Model file for the job. Use its own axes, mm. Face numbers are marked on the shaded views. A direction names the side the tool comes from. Coordinates: 2 decimals unless noted, no trailing zeros. Loops run counter-clockwise (first coordinate to the right, second up) from the corner with the lowest first, then second, coordinate; pieces in that order, holes last. Notation, with made-up numbers: M 73,10 L 106,10 A9 cw 106,25 Z; hole C -39.5,9.25 d9. An arc over 180 degrees is marked long. Write item = value, one per line. Start each with the question number.
from build123d import *

# Parameters (mm, degrees)
BOSS_EXTRUDE1_DEPTH = 127
BOSS_EXTRUDE2_START = 101.6
BOSS_EXTRUDE2_DEPTH = 25.4
SKETCH4_W           = 19.05
SKETCH4_H           = 19.05
SKETCH4_W_2         = 12.7
SKETCH4_H_2         = 12.7
BOSS_EXTRUDE3_DEPTH = 76.2


with BuildPart() as part:
    # Sketch1 → Boss-Extrude1 (new, symmetric)
    with BuildSketch(Plane(origin=(0, 0, 0), x_dir=(0, 0, -1), z_dir=(1, 0, 0))):
        Polygon((0, 0), (0, 51.214865967), (76.2, 51.214865967), (28.702, 0), align=None)
    extrude(amount=BOSS_EXTRUDE1_DEPTH, both=True)

    # Sketch3 → Boss-Extrude2 (add)
    with BuildSketch(Plane(origin=(0, 0, 0), x_dir=(0, 0, -1), z_dir=(1, 0, 0)).offset(BOSS_EXTRUDE2_START)):
        Polygon((0, 51.214865967), (-25.360599441, 0), (0, 0), align=None)
    boss_extrude2 = extrude(amount=BOSS_EXTRUDE2_DEPTH)

    # Mirror1: Boss-Extrude2 across plane
    add(boss_extrude2.mirror(Plane(origin=(0, 0, 0), x_dir=(0, 0, 1), z_dir=(1, 0, 0))))

    # Sketch4 → Boss-Extrude3 (add)
    with BuildSketch(Plane.XY):
        with Locations((114.3, 25.607432983)):
            Rectangle(SKETCH4_W, SKETCH4_H)
        with Locations((114.3, 25.607432983)):
            Rectangle(SKETCH4_W_2, SKETCH4_H_2, mode=Mode.SUBTRACT)
    boss_extrude3 = extrude(amount=BOSS_EXTRUDE3_DEPTH)

    # Mirror2: Boss-Extrude3 across plane
    add(boss_extrude3.mirror(Plane(origin=(0, 0, 0), x_dir=(0, 0, 1), z_dir=(1, 0, 0))))


solid = part.part
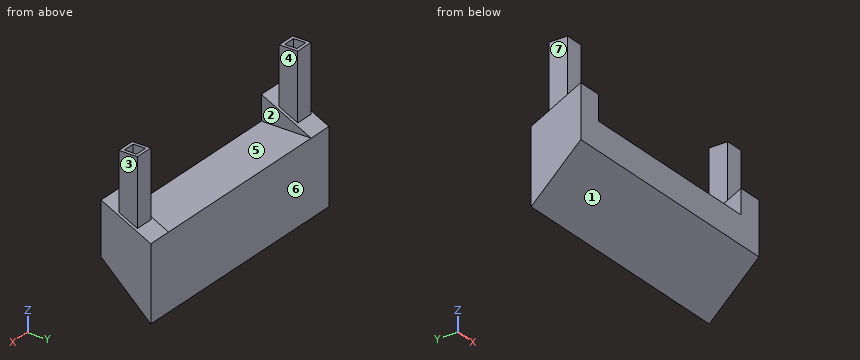
Item 1: Pin check, flat tips, straight feed: pin 1 Ø4 at (x, z) = (111.5, 40) entering from -Y; pin 2 Ø5.5 at (y, z) = (27.5, 52.5) entering from -X (3 decimals); pin 3 Ø4 at (x, z) = (-51, -39) entering from -Y. Stop position of each tip, or through.
Item 2: Cut at C-C (y = 26). Give the cut face in (x, z) (3 decimals), plus the area to 3 significant figures.
Item 3: Pull direction X, two halves, no side cores. Call the marked faces 5, 6 and 7: +X half, -X half, draft (parallel to the pull), parting line (faces both ways), or undercut.
Item 4: Cut at A-A (z = 47). Give the cut face in (x, y) (3 decimals).
Item 5: Probe L1, parallel to X at y = 23, z = 44 (3 decimals); L2, parallel to X at y = 34.5, z = 25 (3 decimals); L3, parallel to X at y = 11.5, z = 15.5. List the from-to ranges inside material, lowest first.
Item 6: Cut at B-B (x = 111.5). Give the cut face in (y, z).
Item 7: Cut at D-D (x = -10.5). Give the cut face in (y, z), plus the area to 3 significant figures.
Item 8: 3-axis set-ups, long thin cutter, end or side, ignore diameter. For the marked faces 1, 2, 3 and 4: which of +Z, -Z, +X, -X, +Y, -Y reach the whole face in a straight line?
Reported:
q1.pin_1 = 16.08
q1.pin_2 = -123.825
q1.pin_3 = 8.95
q2.outline = M -127,-52.815 L 127,-52.815 L 127,12.486 L 123.825,12.486 L 123.825,76.2 L 120.65,76.2 L 120.65,12.486 L 107.95,12.486 L 107.95,76.2 L 104.775,76.2 L 104.775,12.486 L 101.6,12.486 L 101.6,0 L -101.6,0 L -101.6,12.486 L -104.775,12.486 L -104.775,76.2 L -107.95,76.2 L -107.95,12.486 L -120.65,12.486 L -120.65,76.2 L -123.825,76.2 L -123.825,12.486 L -127,12.486 Z
q2.area = 14,900 mm^2
q3.face_5 = undercut
q3.face_6 = draft
q3.face_7 = -X half
q4.outline = M -123.825,16.082 L -104.775,16.082 L -104.775,35.132 L -123.825,35.132 Z; M 104.775,16.082 L 123.825,16.082 L 123.825,35.132 L 104.775,35.132 Z; hole M -120.65,19.257 L -107.95,19.257 L -107.95,31.957 L -120.65,31.957 Z; hole M 107.95,19.257 L 120.65,19.257 L 120.65,31.957 L 107.95,31.957 Z
q5.L1 = -123.825 to -120.65, -107.95 to -104.775, 104.775 to 107.95, 120.65 to 123.825
q5.L2 = -123.825 to -104.775, 104.775 to 123.825
q5.L3 = -127 to -101.6, 101.6 to 127
q6.outline = M 0,-28.7 L 51.21,-76.2 L 51.21,0 L 35.13,7.96 L 35.13,76.2 L 31.96,76.2 L 31.96,9.54 L 19.26,15.82 L 19.26,76.2 L 16.08,76.2 L 16.08,17.4 L 0,25.36 Z
q7.outline = M 0,-28.7 L 51.21,-76.2 L 51.21,0 L 0,0 Z
q7.area = 2,690 mm^2
q8.face_1 = -Z, +X, -X, -Y
q8.face_2 = +Z, +Y, -Y
q8.face_3 = +Z, +X, +Y
q8.face_4 = +Z, +Y
